Here's how the part is built. I have some questions about the finished solid (model axes, mm). A direction names the side the tool comes from. Round coordinates to 2 decimals unless told otherwise and drop trailing zeros. Order: outer loops, then holes, each group sorted by start corner. A loop starts at its lowest first (then second) coordinate and runs counter-clockwise, first axis right, second up. Notation, with made-up numbers: (55.5, 20.25) - (78.5, 20.25) arc R26 ccw to (78.5, 35.25) - close; hole circle Ø11 at (62, -28.5). An arc over 180 degrees is marked (long way). Answer as a JSON object with one key per item and string values.
```python
from build123d import *

# Parameters (mm, degrees)
DODANIE_WYCI_GNI_CIE1_DEPTH = 900
SKORUPA1_T                  = -10
SZKIC4_R                    = 12
DODANIE_WYCI_GNI_CIE3_DEPTH = 15
SZKIC6_R                    = 12.5
SZKIC6_R_2                  = 8.15
DODANIE_WYCI_GNI_CIE4_DEPTH = 10
ZAOKR_GLENIE3_R             = 45
SZKIC8_R                    = 20
WYTNIJ_WYCI_GNI_CIE1_DEPTH  = 7.5
SZKIC11_R                   = 20
WYTNIJ_WYCI_GNI_CIE2_DEPTH  = 5
SZKIC12_R                   = 20
WYTNIJ_WYCI_GNI_CIE3_DEPTH  = 5
SZKIC13_R                   = 20
WYTNIJ_WYCI_GNI_CIE4_DEPTH  = 7.5
ZAOKR_GLENIE4_R             = 10
ZAOKR_GLENIE5_R             = 10


with BuildPart() as part:
    # Szkic1 → Dodanie-wyciągnięcie1 (new body)
    with BuildSketch(Plane.XY):
        with BuildLine():
            Line((-469.846310393, -171.010071663), (0, 0))
            Line((0, 0), (0, -500))
            ThreePointArc((0, -500), (-286.788218176, -409.576022144), (-469.846310393, -171.010071663))
        make_face()
    extrude(amount=DODANIE_WYCI_GNI_CIE1_DEPTH)

    # Skorupa1
    skorupa1_openings = [part.faces().sort_by_distance(p)[0] for p in [
        (-179.521279962, -256.382958146, 900),
        (-179.521279962, -256.382958146, 0),
        (-234.923155196, -85.505035831, 450),
        (0, -250, 450),
    ]]
    offset(amount=SKORUPA1_T, openings=skorupa1_openings, kind=Kind.INTERSECTION)

    # Szkic4 → Dodanie-wyciągnięcie3 (add)
    with BuildSketch(Plane(origin=(0, 0, 0), x_dir=(-1, 0, 0), z_dir=(0, 0, -1))):
        with BuildLine():
            Line((0, -20), (0, -490))
            ThreePointArc((0, -490), (281.052453812, -401.384501702), (460.449384185, -167.58987023))
            Line((460.449384185, -167.58987023), (18.793852416, -6.840402867))
            ThreePointArc((18.793852416, -6.840402867), (-11.471528727, 16.383040886), (0, -20))
        make_face()
        Circle(SZKIC4_R, mode=Mode.SUBTRACT)
    dodanie_wyci_gni_cie3 = extrude(amount=-DODANIE_WYCI_GNI_CIE3_DEPTH)

    # Lustro1: Dodanie-wyciągnięcie3 across plane
    add(dodanie_wyci_gni_cie3.mirror(Plane.XY.offset(450)))

    # Szkic6 → Dodanie-wyciągnięcie4 (add)
    with BuildSketch(Plane.XY.offset(440)):
        with BuildLine():
            Line((-18.793852416, -6.840402867), (-460.449384185, -167.58987023))
            ThreePointArc((-460.449384185, -167.58987023), (-281.052453812, -401.384501702), (0, -490))
            Line((0, -490), (0, -20))
            ThreePointArc((0, -20), (11.471528727, 16.383040886), (-18.793852416, -6.840402867))
        make_face()
        Circle(SZKIC6_R, mode=Mode.SUBTRACT)
        with Locations((-180.698070908, -87.052274649)):
            Circle(SZKIC6_R_2, mode=Mode.SUBTRACT)
        with BuildLine():
            Line((-20, -28.562960135), (-20, -469.574275275))
            ThreePointArc((-20, -469.574275275), (-269.580925085, -385.001460816), (-434.41507852, -179.397713347))
            Line((-434.41507852, -179.397713347), (-199.491923324, -93.892677516))
            ThreePointArc((-199.491923324, -93.892677516), (-173.857668042, -105.846127065), (-161.904218492, -80.211871783))
            Line((-161.904218492, -80.211871783), (-20, -28.562960135))
        make_face(mode=Mode.SUBTRACT)
    dodanie_wyci_gni_cie4 = extrude(amount=-DODANIE_WYCI_GNI_CIE4_DEPTH)

    # Lustro6: Dodanie-wyciągnięcie4 across plane
    add(dodanie_wyci_gni_cie4.mirror(Plane.XY.offset(450)))

    # Zaokrąglenie3
    zaokr_glenie3_edges = [part.edges().sort_by_distance(p)[0] for p in [
        (-434.41507852, -179.397713347, 435),
        (-20, -28.562960135, 435),
        (-20, -469.574275275, 435),
        (-20, -469.574275275, 465),
        (-20, -28.562960135, 465),
        (-434.41507852, -179.397713347, 465),
    ]]
    fillet(zaokr_glenie3_edges, radius=ZAOKR_GLENIE3_R)

    # Szkic8 → Wytnij-wyciągnięcie1 (cut)
    with BuildSketch(Plane(origin=(0, 0, 0), x_dir=(-1, 0, 0), z_dir=(0, 0, -1))):
        Circle(SZKIC8_R)
    extrude(amount=-WYTNIJ_WYCI_GNI_CIE1_DEPTH, mode=Mode.SUBTRACT)

    # Szkic11 → Wytnij-wyciągnięcie2 (cut)
    with BuildSketch(Plane(origin=(0, 0, 430), x_dir=(-1, 0, 0), z_dir=(0, 0, -1))):
        Circle(SZKIC11_R)
    extrude(amount=-WYTNIJ_WYCI_GNI_CIE2_DEPTH, mode=Mode.SUBTRACT)

    # Szkic12 → Wytnij-wyciągnięcie3 (cut)
    with BuildSketch(Plane(origin=(0, 0, 460), x_dir=(-1, 0, 0), z_dir=(0, 0, -1))):
        Circle(SZKIC12_R)
    extrude(amount=-WYTNIJ_WYCI_GNI_CIE3_DEPTH, mode=Mode.SUBTRACT)

    # Szkic13 → Wytnij-wyciągnięcie4 (cut)
    with BuildSketch(Plane(origin=(0, 0, 885), x_dir=(-1, 0, 0), z_dir=(0, 0, -1))):
        Circle(SZKIC13_R)
    extrude(amount=-WYTNIJ_WYCI_GNI_CIE4_DEPTH, mode=Mode.SUBTRACT)

    # Zaokrąglenie4
    zaokr_glenie4_edges = [part.edges().sort_by_distance(p)[0] for p in [
        (-18.793852416, -6.840402867, 437.5),
        (-18.793852416, -6.840402867, 896.25),
        (-18.793852416, -6.840402867, 11.25),
        (-18.793852416, -6.840402867, 467.5),
    ]]
    fillet(zaokr_glenie4_edges, radius=ZAOKR_GLENIE4_R)

    # Zaokrąglenie5
    zaokr_glenie5_edges = [part.edges().sort_by_distance(p)[0] for p in [
        (-199.491923324, -93.892677516, 435),
        (-161.904218492, -80.211871783, 435),
        (-161.904218492, -80.211871783, 465),
        (-199.491923324, -93.892677516, 465),
    ]]
    fillet(zaokr_glenie5_edges, radius=ZAOKR_GLENIE5_R)


solid = part.part
```
1. Imagine slicing it at A-A (y = -298.5). List the corners of the cut face in (x, z) for me, plus the area to 3 significant figures.
Responses:
{"outline": "(-401.12, 0) - (0, 0) - (0, 15) - (-388.58, 15) - (-388.58, 430) - (-363.04, 430) - (-363.04, 440) - (-388.58, 440) - (-388.58, 460) - (-363.04, 460) - (-363.04, 470) - (-388.58, 470) - (-388.58, 885) - (0, 885) - (0, 900) - (-401.12, 900) - close; (-20, 430) - (0, 430) - (0, 440) - (-20, 440) - close; (-20, 460) - (0, 460) - (0, 470) - (-20, 470) - close", "area": "23,900 mm2"}
2. For faces 1 (the face through (-283.28, -412.01, 443.7)), 2 (the face through (-298.817, -130.044, 464.93)), 3 (the face through (-163, -231, 15)), which set-ups out of +Z, -Z, +X, -X, +Y, -Y let a thin tool reach every point of the face, with its end or its side?
Responses:
{"face 1": "+Z, -Z, -X, -Y", "face 2": "none", "face 3": "+X, +Y"}
3. Imagine slicing it at C-C (z = 320). List the corners of the cut face in (x, y) for me, plus the area to 3 significant figures.
Responses:
{"outline": "(-469.85, -171.01) arc R500 ccw to (0, -500) - (0, -490) arc R490 cw to (-460.45, -167.59) - close", "area": "6,050 mm2"}
4. Thinking about a two-plate mould opening in Z: for faces 4 (the face through (13.6, 14.665, 11.198)), 5 (the face through (-8.1, 9.2, 7.5)), 6 (the face through (-231, -104, 430)), which applies, pulls with the +Z half, pulls with the -Z half, needs draft (parallel to the pull), parting line crosses it, or undercut?
Responses:
{"face 4": "needs draft", "face 5": "pulls with the -Z half", "face 6": "undercut"}
5. Imagine slicing it at B-B (x = -230). List the corners of the cut face in (y, z) for me.
Responses:
{"outline": "(-443.96, 0) - (-83.71, 0) - (-83.71, 15) - (-432.67, 15) - (-432.67, 430) - (-409.88, 430) - (-409.88, 440) - (-432.67, 440) - (-432.67, 460) - (-409.88, 460) - (-409.88, 470) - (-432.67, 470) - (-432.67, 885) - (-83.71, 885) - (-83.71, 900) - (-443.96, 900) - close; (-105, 430) - (-83.71, 430) - (-83.71, 440) - (-105, 440) - close; (-105, 460) - (-83.71, 460) - (-83.71, 470) - (-105, 470) - close"}
6. If I drill on L1, parallel to Z at x = -7.5, y = -389; L2, parallel to Z at x = -90.5, y = -214; L3, parallel to Y at x = -5.5, z = 356, over which ranges is the centre line in solid material (lowest first)? Write a range as [from, to].
Responses:
{"L1": "[0, 15], [430, 440], [460, 470], [885, 900]", "L2": "[0, 15], [885, 900]", "L3": "[-499.97, -489.97]"}
7. For P1, Ø2, axis at x = -230.5, z = 714.5, coming from the +Y side; P2, Ø10, axis at x = -284, z = 708.5, coming from the -Y side; P3, Ø20, axis at x = -8, y = 3.5, coming from the -Z side, each with a flat end and sliding along its axis, tell me the tip position at first contact or that it passes through.
Responses:
{"P1": "y = -431.87", "P2": "y = -414.92", "P3": "z = 7.5"}
